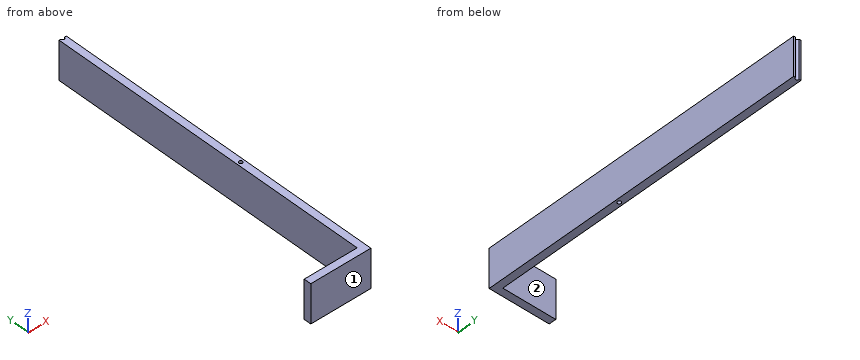
from build123d import *

# Parameters (mm, degrees)
SZKIC2_W                   = 130
SZKIC2_H                   = 24
SZKIC3_R                   = 6
WYTNIJ_WYCI_GNI_CIE1_DEPTH = 131


with BuildPart() as part:
    # Wyciągnięcie po ścieżce1: sweep along a path in Szkic1
    with BuildLine(Plane.XY) as wyci_gni_cie_po_cie_ce1_path:
        Line((0, 0), (190, 0))
        Line((190, 0), (190, 1100))
    # Szkic2 → Wyciągnięcie po ścieżce1 (sweep)
    with BuildSketch(Plane(origin=(0, 0, 0), x_dir=(0, 0, -1), z_dir=(1, 0, 0))):
        Rectangle(SZKIC2_W, SZKIC2_H)
    sweep(path=wyci_gni_cie_po_cie_ce1_path.line, transition=Transition.RIGHT)

    # Szkic3 → Wytnij-wyciągnięcie1 (cut, through all)
    with BuildSketch(Plane.XY.offset(65)):
        with Locations((190, 1100)):
            Circle(SZKIC3_R)
        with Locations((190, 450)):
            Circle(SZKIC3_R)
    extrude(amount=-WYTNIJ_WYCI_GNI_CIE1_DEPTH, mode=Mode.SUBTRACT)


solid = part.part
Source: CAD feature listing. Evaluate the final solid. Frame: model axes, mm. Face numbers are marked on the shaded views. A direction names the side the tool comes from. Coordinates: 2 decimals unless noted, no trailing zeros. Loops run counter-clockwise (first coordinate to the right, second up) from the corner with the lowest first, then second, coordinate; pieces in that order, holes last. Notation, with made-up numbers: (3.5, -17.5) -> (12.5, -17.5) arc R32 ccw to (12.5, 10.5) -> close; hole circle Ø4 at (7, 78.5). An arc over 180 degrees is marked (long way). Answer in a Markdown table with one row per item. Add a question column.
Q1. Section B-B on y = 771.5. Return the cut outline in (x, z), and give its area (3 significant figures).
Q2. Contact query for flat-ended pins moving along their axis: pin 1 Ø12 at (y, z) = (898, 12) entering from -X; pin 2 Ø1.5 at (x, z) = (94.5, -27.5) entering from +Y. Output: stop coordinate, or through.
Q3. Ray query, line 1 along X through (y, z) = (450, 35); line 2 along Y through (x, z) = (190, 12); line 3 along X through (y, z) = (576.5, -25.5). Return the intervals inside material, ascending.
Q4. Section C-C on x = 118.5. Return the cut outline in (y, z).
Q5. Reachability of the marked faces 1 and 2 from +Z, -Z, +X, -X, +Y, -Y: full face, straight path, thin tool, end or side. Return the list, or none.
Q6. Section A-A on z = 10. Return the cut outline in (x, y).
Computed values:
| question | item | result |
|---|---|---|
| 1 | outline | (178, -65) -> (202, -65) -> (202, 65) -> (178, 65) -> close |
| 1 | area | 3,120 mm^2 |
| 2 | pin 1 | stops at x = 178 |
| 2 | pin 2 | stops at y = 12 |
| 3 | line 1 | x = 178 to 184, 196 to 202 |
| 3 | line 2 | y = -12 to 444, 456 to 1094 |
| 3 | line 3 | x = 178 to 202 |
| 4 | outline | (-12, -65) -> (12, -65) -> (12, 65) -> (-12, 65) -> close |
| 5 | face 1 | +Z, -Z, +X, -X, -Y |
| 5 | face 2 | +Z, -Z, -X, +Y |
| 6 | outline | (0, -12) -> (202, -12) -> (202, 1100) -> (196, 1100) arc R6 cw to (184, 1100) -> (178, 1100) -> (178, 12) -> (0, 12) -> close; hole circle Ø12 at (190, 450) |
